The listing builds one solid part. Answer for the finished solid, in the listing's coordinates (mm). Face numbers are marked on the shaded views. Coordinates: 2 decimals unless noted, no trailing zeros. Order: outer loops, then holes, each group sorted by start corner. A loop starts at its lowest first (then second) coordinate and runs counter-clockwise, first axis right, second up. Notation, with made-up numbers: (-24.5, 66.5) - (2.5, 66.5) arc R20 ccw to (2.5, 75.5) - close; hole circle Ø10 at (-27.5, 29.25). An arc over 180 degrees is marked (long way). Use a Markdown table: item, result. Add a question column.
Item 1: Flat-ended cylindrical pins translate along their axes: P1, Ø3, axis at y = -11.5, z = 4, coming from the -X side; P2, Ø3, axis at y = -13, z = 1.5, coming from the -X side. Find the tip coordinate at first contact, or state that the pin passes through.
Item 2: The part is cut by section C-C, the plane z = 1.3. Give the vertices of the cut face in (x, y), then the cut area to 3 significant figures.
Item 3: The part is cut by section A-A, the plane x = 0. Give the vertices of the cut face in (y, z), then the cut area to 3 significant figures.
Item 4: The part is cut by section B-B, the plane y = -13.45. Give the vertices of the cut face in (x, z).
Item 5: Find the intervals of material crossed by line 1 along Y through (x, z) = (0, 1.15); line 2 along Y through (x, z) = (7.5, 3.8); line 3 along X through (y, z) = (-14, 0.35), in increasing order.
Item 6: The mould has two halves that part along Y. Classify the marked faces 1, 2 and 3: released by +Y, released by -Y, zero draft, split by the parting line, or undercut.
Item 7: The part is cut by section D-D, the plane x = -10.25. Give the vertices of the cut face in (y, z), then the cut area to 3 significant figures.
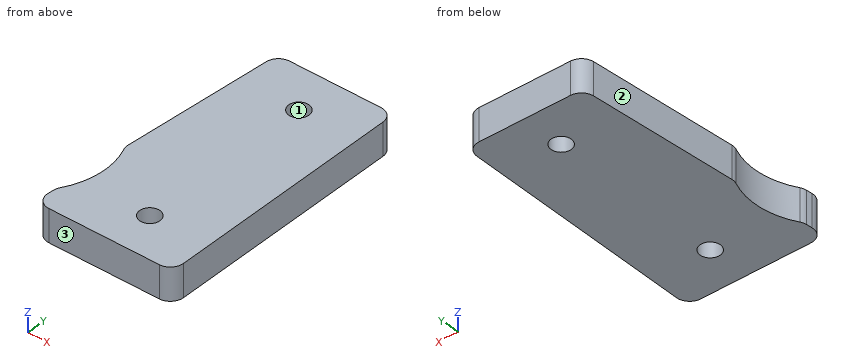
from build123d import *

# Parameters (mm, degrees)
SKETCH_1_W               = 30
SKETCH_1_H               = 40
EXTRUDE_1_DEPTH          = 5
CUT_EXTRUDE_1_DEPTH      = 800
SKETCH_3_R               = 1.55
CUT_EXTRUDE_2_DEPTH      = 10
FILLET_1_R               = 2
SKETCH_4_R               = 11.5
CUT_EXTRUDE_3_DEPTH      = 10
FILLET_2_R               = 2
CUT_EXTRUDE_5_DEPTH      = 26.495097568
CUT_EXTRUDE_5_DEPTH_BACK = 5
FILLET_4_R               = 2


with BuildPart() as part:
    # 草图1 → 凸台-拉伸1 (new body)
    with BuildSketch(Plane.XY):
        Rectangle(SKETCH_1_W, SKETCH_1_H)
    extrude(amount=EXTRUDE_1_DEPTH)

    # 草图2 → 切除-拉伸1 (cut)
    with BuildSketch(Plane.XY.offset(5)):
        Polygon((-8.819854033, 20), (-12.017512264, -20), (-15, -20), (-15, 20), align=None)
    extrude(amount=-CUT_EXTRUDE_1_DEPTH, mode=Mode.SUBTRACT)

    # 草图3 → 切除-拉伸2 (cut)
    with BuildSketch(Plane.XY.offset(5)):
        with Locations((0, 13.45)):
            Circle(SKETCH_3_R)
        with Locations((0, -13.45)):
            Circle(SKETCH_3_R)
    extrude(amount=-CUT_EXTRUDE_2_DEPTH, mode=Mode.SUBTRACT)

    # 圆角1
    fillet_1_edges = [part.edges().sort_by_distance(p)[0] for p in [
        (-12.017512264, -20, 2.5),
        (-8.819854033, 20, 2.5),
        (15, -20, 2.5),
        (15, 20, 2.5),
    ]]
    fillet(fillet_1_edges, radius=FILLET_1_R)

    # 草图4 → 切除-拉伸3 (cut)
    with BuildSketch(Plane.XY.offset(5)):
        with Locations((-21.25, -10)):
            Circle(SKETCH_4_R)
    extrude(amount=-CUT_EXTRUDE_3_DEPTH, mode=Mode.SUBTRACT)

    # 圆角2
    fillet_2_edges = [part.edges().sort_by_distance(p)[0] for p in [
        (-11.734337347, -16.457721291, 2.5),
        (-10.829264337, -5.136023413, 2.5),
    ]]
    fillet(fillet_2_edges, radius=FILLET_2_R)

    # 草图6 → 切除-拉伸5 (cut, two sides: drawn at the far end of the back side and taken through both)
    with BuildSketch(Plane.XY.offset(5).offset(-CUT_EXTRUDE_5_DEPTH_BACK)):
        Polygon((9, 120.21695141), (9, 20), (9, -20), (9, -120.21695141), (209.433902819, -120.21695141), (209.433902819, 120.21695141), align=None)
    extrude(amount=CUT_EXTRUDE_5_DEPTH + CUT_EXTRUDE_5_DEPTH_BACK, mode=Mode.SUBTRACT)

    # 圆角4
    fillet_4_edges = [part.edges().sort_by_distance(p)[0] for p in [
        (9, 20, 2.5),
        (9, -20, 2.5),
    ]]
    fillet(fillet_4_edges, radius=FILLET_4_R)


solid = part.part
Solution:
| question | item | result |
|---|---|---|
| 1 | P1 | stops at x = -10.15 |
| 1 | P2 | stops at x = -10.67 |
| 2 | outline | (-11.84, -17.84) arc R2 ccw to (-9.85, -20) - (7, -20) arc R2 ccw to (9, -18) - (9, 18) arc R2 ccw to (7, 20) - (-6.97, 20) arc R2 ccw to (-8.97, 18.16) - (-10.79, -4.63) arc R2 ccw to (-10.64, -5.56) arc R11.5 cw to (-11.48, -16.07) arc R2 ccw to (-11.77, -16.96) - close; hole circle Ø3.1 at (0, -13.45); hole circle Ø3.1 at (0, 13.45) |
| 2 | area | 747 mm2 |
| 3 | outline | (-20, 0) - (-15, 0) - (-15, 5) - (-20, 5) - close; (-11.9, 0) - (11.9, 0) - (11.9, 5) - (-11.9, 5) - close; (15, 0) - (20, 0) - (20, 5) - (15, 5) - close |
| 3 | area | 169 mm2 |
| 4 | outline | (-10.28, 0) - (-1.55, 0) - (-1.55, 5) - (-10.28, 5) - close; (1.55, 0) - (9, 0) - (9, 5) - (1.55, 5) - close |
| 5 | line 1 | y = -20 to -15, -11.9 to 11.9, 15 to 20 |
| 5 | line 2 | y = -19.94 to 19.94 |
| 5 | line 3 | x = -10.47 to -1.45, 1.45 to 9 |
| 6 | face 1 | undercut |
| 6 | face 2 | released by +Y |
| 6 | face 3 | released by -Y |
| 7 | outline | (-19.96, 0) - (-13.35, 0) - (-13.35, 5) - (-19.96, 5) - close; (-6.65, 0) - (2.11, 0) - (2.11, 5) - (-6.65, 5) - close |
| 7 | area | 76.8 mm2 |
